Part model, mm, in its own coordinate system. A direction names the side the tool comes from. Round coordinates to 2 decimals unless told otherwise and drop trailing zeros. Loops run counter-clockwise (first coordinate to the right, second up) from the corner with the lowest first, then second, coordinate; pieces in that order, holes last. Notation, with made-up numbers: (-26.75, 48.25) - (2.25, 48.25) arc R27 cw to (2.25, 87.25) - close; hole circle Ø4 at (26, -9). An arc over 180 degrees is marked (long way). Write each question's results on one line, items separated by ' | '. Start each with the question number.
(1) Tool access for faces 1 (the face through (160, -443, 0)), 2 (the face through (126, -504.896, 3)), 3 (the face through (-104.8, -419.35, -129.5)), 4 (the face through (-84.5, -456, -57)), 5 (the face through (-104.8, -409.35, -129.5)): list every direction of +Z, -Z, +X, -X, +Y, -Y with a clear straight run to the whole face (end or side of a thin tool).
(2) Cut at B-B, the plane x = 127. List the corners of the cut face in (y, z), then the cut area to 3 significant figures.
(3) Flat gauge pins, fed straight in: P1, Ø16.5, axis at x = -115.5, z = -20.5, coming from the -Y side; P2, Ø11.5, axis at x = -104, z = -134, coming from the +Y side; P3, Ø3, axis at x = -114.5, y = -412, coming from the -Z side. Where does each tip first touch, or does it go through?
(4) Drill centre lines: L1, parallel to X at y = -364, z = 3; L2, parallel to Y at x = -41, z = 2.05; L3, parallel to X at y = -406.5, z = -69.5. Where is each one in solid material? Low to high.
(5) Cut at C-C, the plane y = -400. List the corners of the cut face in (x, z), then the cut area to 3 significant figures.
(6) Mould opens along Z. For faces 6 (the face through (-1, -424, 0)), 7 (the face through (-109, -495, -106.226)), 8 (the face through (-104.8, -490.377, -129.5)) say: released by +Z, released by -Z, zero draft, split by the parting line, or undercut.
(7) Cut at A-A, the plane z = -94. List the corners of the cut face in (x, y), then the cut area to 3 significant figures.
from build123d import *

# Parameters (mm, degrees)
CROQUIS1_R              = 7
CROQUIS1_R_2            = 5.25
CROQUIS1_R_3            = 5
CROQUIS1_R_4            = 8
SALIENTE_EXTRUIR1_DEPTH = 5
CROQUIS2_W              = 5
CROQUIS2_H              = 100
SALIENTE_EXTRUIR2_DEPTH = 100
CROQUIS3_W              = 5
CROQUIS3_H              = 20
SALIENTE_EXTRUIR3_DEPTH = 50
CROQUIS4_W              = 37.618444679
CROQUIS4_H              = 10
SALIENTE_EXTRUIR4_DEPTH = 40
CROQUIS5_R              = 7
CORTAR_EXTRUIR1_DEPTH   = 325.287034049
NERVIO1_REACH           = 304.992
CROQUIS6_WALL_W         = 701.273547134
CROQUIS6_WALL_H         = 10
NERVIO2_REACH           = 304.992
CROQUIS7_WALL_W         = 718.906485388
CROQUIS7_WALL_H         = 10


with BuildPart() as part:
    # Croquis1 → Saliente-Extruir1 (new body)
    with BuildSketch(Plane.XY):
        with BuildLine():
            Line((232.166801748, -404.895674081), (84.5, -404.895674081))
            Line((84.5, -404.895674081), (84.5, -330.787715528))
            Line((84.5, -330.787715528), (-84.5, -330.787715528))
            Line((-84.5, -330.787715528), (-84.5, -404.895674081))
            Line((-84.5, -404.895674081), (-175.19051762, -404.895674081))
            ThreePointArc((-175.19051762, -404.895674081), (-225.19051762, -454.895674081), (-175.19051762, -504.895674081))
            Line((-175.19051762, -504.895674081), (-84.5, -504.895674081))
            Line((-84.5, -504.895674081), (-84.5, -520))
            Line((-84.5, -520), (84.5, -520))
            Line((84.5, -520), (84.5, -504.895674081))
            Line((84.5, -504.895674081), (232.166801748, -504.895674081))
            Line((232.166801748, -504.895674081), (232.166801748, -404.895674081))
        make_face()
        with Locations((-175.19051762, -454.895674081)):
            Circle(CROQUIS1_R, mode=Mode.SUBTRACT)
        with Locations((41, -364.3)):
            Circle(CROQUIS1_R_2, mode=Mode.SUBTRACT)
        with Locations((-41, -364.3)):
            Circle(CROQUIS1_R_2, mode=Mode.SUBTRACT)
        with Locations((47, -485)):
            Circle(CROQUIS1_R_3, mode=Mode.SUBTRACT)
        with Locations((-47, -485)):
            Circle(CROQUIS1_R_3, mode=Mode.SUBTRACT)
        with Locations((212.922919346, -454.766206892)):
            Circle(CROQUIS1_R_4, mode=Mode.SUBTRACT)
    extrude(amount=SALIENTE_EXTRUIR1_DEPTH)

    # Croquis2 → Saliente-Extruir2 (add)
    with BuildSketch(Plane(origin=(0, 0, 0), x_dir=(-1, 0, 0), z_dir=(0, 0, -1))):
        with Locations((-87, -454.895674081)):
            Rectangle(CROQUIS2_W, CROQUIS2_H)
        with Locations((87, -454.895674081)):
            Rectangle(CROQUIS2_W, CROQUIS2_H)
    extrude(amount=SALIENTE_EXTRUIR2_DEPTH)

    # Croquis3 → Saliente-Extruir3 (add)
    with BuildSketch(Plane(origin=(0, 0, -100), x_dir=(-1, 0, 0), z_dir=(0, 0, -1))):
        with Locations((87, -494.895674081)):
            Rectangle(CROQUIS3_W, CROQUIS3_H)
        with Locations((87, -414.895674081)):
            Rectangle(CROQUIS3_W, CROQUIS3_H)
    extrude(amount=SALIENTE_EXTRUIR3_DEPTH)

    # Croquis4 → Saliente-Extruir4 (add)
    with BuildSketch(Plane.ZY.offset(89.5)):
        with Locations((-125.035404741, -414.350039231)):
            Rectangle(CROQUIS4_W, CROQUIS4_H)
        with Locations((-125.035404741, -495.377386848)):
            Rectangle(CROQUIS4_W, CROQUIS4_H)
    extrude(amount=SALIENTE_EXTRUIR4_DEPTH)

    # Croquis5 → Cortar-Extruir1 (cut, through all)
    with BuildSketch(Plane.XZ.offset(500.377386848)):
        with Locations(Location((-110.45279813, -124.886599464, 0), (0, 0, 270))):
            Circle(CROQUIS5_R)
    extrude(amount=-CORTAR_EXTRUIR1_DEPTH, mode=Mode.SUBTRACT)

    # Croquis6 wall → Nervio1 (add, up to next)
    with BuildSketch(Plane(origin=(-117.239432288, -454.895674081, -37.5), x_dir=(-0.594696602605, 0, 0.803950216649), z_dir=(-0.803950216649, 0, -0.594696602605)), mode=Mode.PRIVATE) as nervio1_sk1:
        Rectangle(CROQUIS6_WALL_W, CROQUIS6_WALL_H)
    nervio1_tool1 = extrude(nervio1_sk1.sketch, amount=-NERVIO1_REACH, mode=Mode.PRIVATE) - part.part
    add(nervio1_tool1.solids().sort_by_distance((-117.239432288, -454.895674081, -37.5))[0])

    # Croquis7 wall → Nervio2 (add, up to next)
    with BuildSketch(Plane(origin=(133.798766553, -454.895674081, -33.37002042), x_dir=(-0.79873511165, 0, -0.601682824599), z_dir=(0.601682824599, 0, -0.79873511165)), mode=Mode.PRIVATE) as nervio2_sk1:
        Rectangle(CROQUIS7_WALL_W, CROQUIS7_WALL_H)
    nervio2_tool1 = extrude(nervio2_sk1.sketch, amount=-NERVIO2_REACH, mode=Mode.PRIVATE) - part.part
    add(nervio2_tool1.solids().sort_by_distance((133.798766553, -454.895674081, -33.37002042))[0])


solid = part.part
A:
1) face 1: -Z, +X | face 2: +Z, -Z, +X, -Y | face 3: -Z, -X | face 4: -Z, +Y, -Y | face 5: -Z, -X, +Y
2) outline: (-504.9, 0) - (-459.9, 0) - (-459.9, -38.49) - (-449.9, -38.49) - (-449.9, 0) - (-404.9, 0) - (-404.9, 5) - (-504.9, 5) - close | area: 885 mm2
3) P1: y = -459.9 | P2: y = -409.35 | P3: z = -143.84
4) L1: -84.5 to -46.24, -35.76 to 35.76, 46.24 to 84.5 | L2: -520 to -369.55, -359.05 to -330.79 | L3: -89.5 to -84.5, 84.5 to 89.5
5) outline: (-84.5, 0) - (84.5, 0) - (84.5, 5) - (-84.5, 5) - close | area: 845 mm2
6) face 6: released by -Z | face 7: undercut | face 8: zero draft
7) outline: (-89.5, -504.9) - (-84.5, -504.9) - (-84.5, -404.9) - (-89.5, -404.9) - close; (84.5, -504.9) - (89.5, -504.9) - (89.5, -404.9) - (84.5, -404.9) - close | area: 1,000 mm2
